Here's how the part is built. I have some questions about the finished solid (model axes, mm). A direction names the side the tool comes from. Round coordinates to 2 decimals unless told otherwise and drop trailing zeros. Write each loop counter-clockwise with the first axis right and the second up, starting at its lowest first coordinate (ties: lowest second). Pieces come first, ordered by that corner, then holes. Notation, with made-up numbers: (5, 89) -> (17, 89) arc R15 ccw to (17, 118) -> close; hole circle Ø9 at (71, 29). An arc over 180 degrees is marked (long way). Answer as CSV lines item,"result".
from build123d import *

# Parameters (mm, degrees)
BOSS_EXTRUDE1_DEPTH = 0.5


with BuildPart() as part:
    # Sketch1 → Boss-Extrude1 (new, symmetric)
    with BuildSketch(Plane.XY):
        with BuildLine():
            Line((22, -10), (-22, -10))
            ThreePointArc((-22, -10), (-23.414213562, -9.414213562), (-24, -8))
            Line((-24, -8), (-24, 8))
            ThreePointArc((-24, 8), (-23.414213562, 9.414213562), (-22, 10))
            Line((-22, 10), (22, 10))
            ThreePointArc((22, 10), (23.414213562, 9.414213562), (24, 8))
            Line((24, 8), (24, -8))
            ThreePointArc((24, -8), (23.414213562, -9.414213562), (22, -10))
        make_face()
        with BuildLine():
            Line((-2.5, -2.5), (-2.5, 2.5))
            ThreePointArc((-2.5, 2.5), (0, 5), (2.5, 2.5))
            Line((2.5, 2.5), (2.5, -2.5))
            ThreePointArc((2.5, -2.5), (0, -5), (-2.5, -2.5))
        make_face(mode=Mode.SUBTRACT)
        with BuildLine():
            Line((-8.5, -3.5), (-8.5, 3.5))
            ThreePointArc((-8.5, 3.5), (-7, 5), (-5.5, 3.5))
            Line((-5.5, 3.5), (-5.5, -3.5))
            ThreePointArc((-5.5, -3.5), (-7, -5), (-8.5, -3.5))
        make_face(mode=Mode.SUBTRACT)
        with BuildLine():
            Line((5.5, -3.5), (5.5, 3.5))
            ThreePointArc((5.5, 3.5), (7, 5), (8.5, 3.5))
            Line((8.5, 3.5), (8.5, -3.5))
            ThreePointArc((8.5, -3.5), (7, -5), (5.5, -3.5))
        make_face(mode=Mode.SUBTRACT)
    extrude(amount=BOSS_EXTRUDE1_DEPTH, both=True)


solid = part.part
Item 1: Suppose I cut it at B-B, the plane y = 1.5. List the corners of the cut face in (x, z) for me, then the cut area to 3 significant figures.
Results found:
outline,"(-24, -0.5) -> (-8.5, -0.5) -> (-8.5, 0.5) -> (-24, 0.5) -> close; (-5.5, -0.5) -> (-2.5, -0.5) -> (-2.5, 0.5) -> (-5.5, 0.5) -> close; (2.5, -0.5) -> (5.5, -0.5) -> (5.5, 0.5) -> (2.5, 0.5) -> close; (8.5, -0.5) -> (24, -0.5) -> (24, 0.5) -> (8.5, 0.5) -> close"
area,"37.0 mm²"
Item 2: Suppose I cut it at A-A, the plane x = 7. List the corners of the cut face in (y, z) for me.
Results found:
outline,"(-10, -0.5) -> (-5, -0.5) -> (-5, 0.5) -> (-10, 0.5) -> close; (5, -0.5) -> (10, -0.5) -> (10, 0.5) -> (5, 0.5) -> close"
Item 3: I need wall thicknesses on L1, parallel to X at y = 1.25, z = -0.3; L2, parallel to X at y = -3, z = 0.15; L3, parallel to X at y = -8.25, z = -0.15. Which ranges of each line are inside material? Lowest first, please.
Results found:
L1,"x = -24 to -8.5, -5.5 to -2.5, 2.5 to 5.5, 8.5 to 24"
L2,"x = -24 to -8.5, -5.5 to -2.45, 2.45 to 5.5, 8.5 to 24"
L3,"x = -23.98 to 23.98"
Item 4: If we mould it in two halves opening along Y, with no side actions, what happens to faces 1 (the flat face through (-24, 0, 0)), 2 (the cylindrical face through (-23.4, -9.43, 0.01)), 3 (the cylindrical face through (0, 5, 0))? For each: pulls with the +Y half, pulls with the -Y half, needs draft (parallel to the pull), parting line crosses it, or undercut.
Results found:
face 1,"needs draft"
face 2,"pulls with the -Y half"
face 3,"undercut"
Item 5: Suppose I cut it at C-C, the plane z = 0.05. List the corners of the cut face in (x, y) for me, then the cut area to 3 significant figures.
Results found:
outline,"(-24, -8) arc R2 ccw to (-22, -10) -> (22, -10) arc R2 ccw to (24, -8) -> (24, 8) arc R2 ccw to (22, 10) -> (-22, 10) arc R2 ccw to (-24, 8) -> close; hole (-8.5, -3.5) arc R1.5 ccw to (-5.5, -3.5) -> (-5.5, 3.5) arc R1.5 ccw to (-8.5, 3.5) -> close; hole (-2.5, -2.5) arc R2.5 ccw to (2.5, -2.5) -> (2.5, 2.5) arc R2.5 ccw to (-2.5, 2.5) -> close; hole (5.5, -3.5) arc R1.5 ccw to (8.5, -3.5) -> (8.5, 3.5) arc R1.5 ccw to (5.5, 3.5) -> close"
area,"856 mm²"
Item 6: For faces 4 (the cylindrical face through (23.43, -9.4, 0.01)), 5 (the flat face through (-5.5, 0, 0)), which set-ups out of +Z, -Z, +X, -X, +Y, -Y let a thin tool reach every point of the face, with its end or its side?
Results found:
face 4,"+Z, -Z, +X, -Y"
face 5,"+Z, -Z"
Item 7: Suppose I cut it at D-D, the plane x = -1.5. List the corners of the cut face in (y, z) for me, then the cut area to 3 significant figures.
Results found:
outline,"(-10, -0.5) -> (-4.5, -0.5) -> (-4.5, 0.5) -> (-10, 0.5) -> close; (4.5, -0.5) -> (10, -0.5) -> (10, 0.5) -> (4.5, 0.5) -> close"
area,"11.0 mm²"
